```python
from build123d import *

# Parameters (mm, degrees)
F0_W     = 0.9
F0_H     = 1.7
F1_DEPTH = 48
F0_W_2   = 6
F0_H_2   = 3
F2_DEPTH = 2
F3_R     = 0.5


with BuildPart() as f1:
    # F0 (on Top) → F1 (new body)
    with BuildSketch(Plane.XY):
        Polygon((-26.985715, 13.8), (-28.785715, 13.8), (-28.785715, 0), (32.814285, 0), (32.814285, 13.8), (31.014285, 13.8), (31.014285, 12.7), (31.014285, 11), (31.014285, 1.8), (-26.985715, 1.8), (-26.985715, 11), (-26.985715, 12.7), align=None)
        with Locations((-26.535715, 11.85)):
            Rectangle(F0_W, F0_H)
        with Locations((30.564285, 11.85)):
            Rectangle(F0_W, F0_H)
    extrude(amount=-F1_DEPTH)

    # F0 (on Top) → F2 (join)
    with BuildSketch(Plane.XY):
        Polygon((31.014285, 13.8), (-26.985715, 13.8), (-26.985715, 12.7), (-26.085715, 12.7), (-26.085715, 11), (-26.985715, 11), (-26.985715, 1.8), (31.014285, 1.8), (31.014285, 11), (30.114285, 11), (30.114285, 12.7), (31.014285, 12.7), align=None)
        with Locations((0, 10.3)):
            Rectangle(F0_W_2, F0_H_2, mode=Mode.SUBTRACT)
        Polygon((-26.985715, 13.8), (-28.785715, 13.8), (-28.785715, 0), (32.814285, 0), (32.814285, 13.8), (31.014285, 13.8), (31.014285, 12.7), (31.014285, 11), (31.014285, 1.8), (-26.985715, 1.8), (-26.985715, 11), (-26.985715, 12.7), align=None)
        with Locations((-26.535715, 11.85)):
            Rectangle(F0_W, F0_H)
        with Locations((30.564285, 11.85)):
            Rectangle(F0_W, F0_H)
    extrude(amount=F2_DEPTH)

    # F3
    f3_edges = [f1.edges().sort_by_distance(p)[0] for p in [
        (-26.535715, 11, -48),
        (-26.535715, 12.7, -48),
        (-26.085715, 11.85, -48),
        (30.564285, 11, -48),
        (30.564285, 12.7, -48),
        (30.114285, 11.85, -48),
    ]]
    fillet(f3_edges, radius=F3_R)


solid = f1.part
```
For this review, take the finished solid that the model builds, in its own axes (mm). A direction names the side the tool comes from. Coordinates: 2 decimals unless noted, no trailing zeros. Order: outer loops, then holes, each group sorted by start corner. A loop starts at its lowest first (then second) coordinate and runs counter-clockwise, first axis right, second up. Notation, with made-up numbers: (22.5, 56) - (70.5, 56) arc R22 ccw to (70.5, 81) - close; hole circle Ø3 at (45, 67). An arc over 180 degrees is marked (long way). Answer as a JSON object with one key per item and string values. Group by question number.
1. We need section C-C on x = -24. State the section outline as (y, z) points.
2. We need section A-A on y = 3.25. State the section outline as (x, z) points, then the cut area to 3 significant figures.
3. For faces 5 (the flat face through (-26.986, 7, -24)), 6 (the flat face through (30.114, 12, -23)), 7 (the flat face through (-3, 10, 1)), list the 3-axis set-ups (+Z, -Z, +X, -X, +Y, -Y) from which the entire face can be reached by the end or side of a thin tool; tool diameter is ignored.
4. For probe 1 along X at (y, z) = (8, -16); probe 2 along Y at (x, z) = (0.5, -18); probe 3 along Z at (x, y) = (-14, 6.25), list the stretches that pass through material, from the lowest coordinate up.
5. The part is to be moulded in two halves that separate along X. For faces 1 (the flat face through (2, 1.8, -24)), 2 (the flat face through (-28.786, 7, -23)), 3 (the flat face through (0, 8.8, 1)), 4 (the flat face through (2, 7, 2)), say which applies: pulls with the +X half, pulls with the -X half, needs draft (parallel to the pull), parting line crosses it, or undercut.
6. Clearance check with flat-ended pins moving along their axes: P1, Ø1.5, axis at x = 3, y = 12, coming from the -Z side; P2, Ø14.5, axis at x = 9, z = -31, coming from the +Y side. State where each tip first meets the part, or that it passes through.
7. We need section B-B on z = -14. State the section outline as (x, y) points.
Final values:
{
 "1": {"outline": "(0, -48) - (1.8, -48) - (1.8, 0) - (13.8, 0) - (13.8, 2) - (0, 2) - close"},
 "2": {"outline": "(-28.79, -48) - (-26.99, -48) - (-26.99, 0) - (31.01, 0) - (31.01, -48) - (32.81, -48) - (32.81, 2) - (-28.79, 2) - close", "area": "296 mm²"},
 "3": {"face 5": "-Z", "face 6": "-Z, +Y", "face 7": "+Z, -Z"},
 "4": {"probe 1": "-28.79 to -26.99, 31.01 to 32.81", "probe 2": "0 to 1.8", "probe 3": "0 to 2"},
 "5": {"face 1": "undercut", "face 2": "pulls with the -X half", "face 3": "undercut", "face 4": "needs draft"},
 "6": {"P1": "z = 0", "P2": "y = 1.8"},
 "7": {"outline": "(-28.79, 0) - (32.81, 0) - (32.81, 13.8) - (31.01, 13.8) - (31.01, 12.7) - (30.11, 12.7) - (30.11, 11) - (31.01, 11) - (31.01, 1.8) - (-26.99, 1.8) - (-26.99, 11) - (-26.09, 11) - (-26.09, 12.7) - (-26.99, 12.7) - (-26.99, 13.8) - (-28.79, 13.8) - close"}
}
